For this review, use the dimensioned drawing (mm, ordinates from the lowest corner) and the shaded views. A direction names the side the tool comes from. Give positions to 0.01 mm unless a question says otherwise; leave off trailing zeros. Write each loop counter-clockwise with the first axis right and the second up, starting at its lowest first coordinate (ties: lowest second). Pieces come first, ordered by that corner, then holes. Notation, with made-up numbers: (30.25, 52) -> (49.25, 52) arc R25 ccw to (49.25, 69) -> close; hole circle Ø11 at (24, 42). An arc over 180 degrees is marked (long way). Return JSON: item names as keys, results as strings.
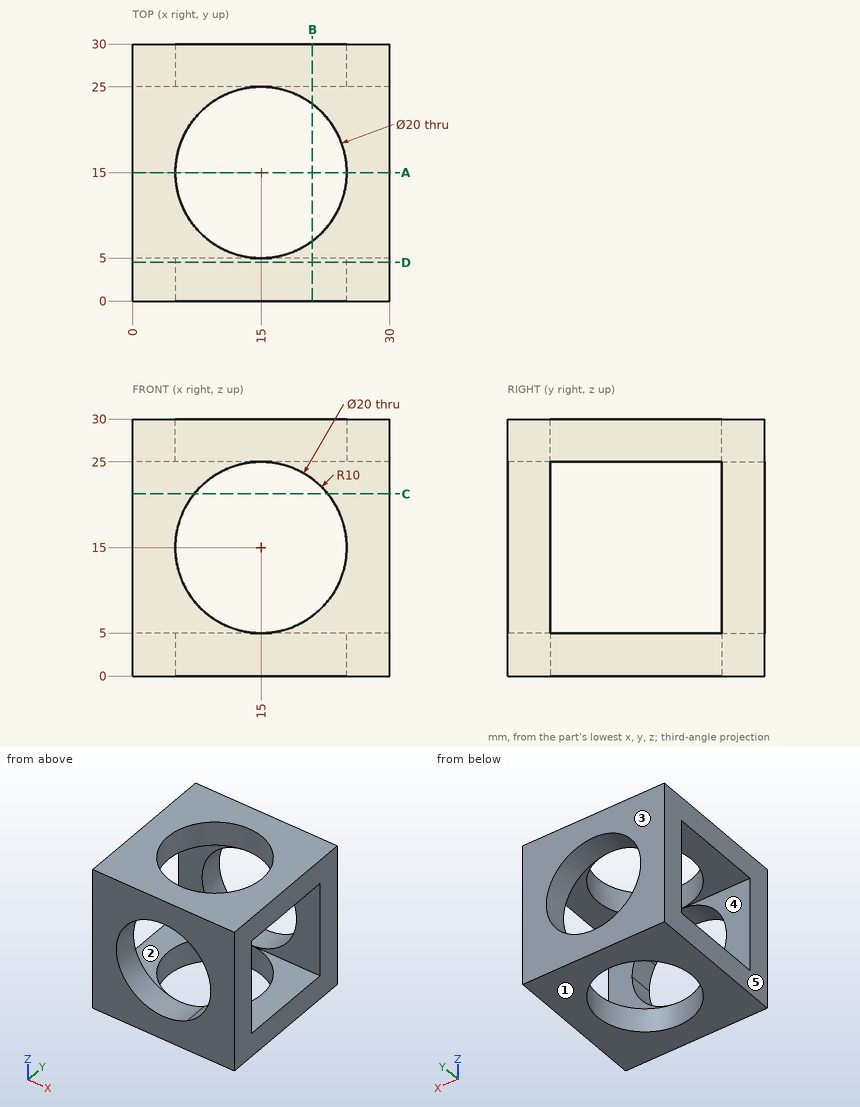
1. For pin 1 (18 mm diameter, centred on x = 15, z = 15, fed in from -Y), flat-tipped, find the tip position at first contact; note if it passes through.
Results found:
{"pin 1": "passes through"}
2. For the marked faces 4 and 5, list the 3-axis set-ups (+Z, -Z, +X, -X, +Y, -Y) from which the entire face can be reached by the end or side of a thin tool; tool diameter is ignored.
Results found:
{"face 4": "+X, -X", "face 5": "+Z, -Z, -X, +Y, -Y"}
3. The part is to be moulded in two halves that separate along Z. For the marked faces 1, 2 and 3, say which applies: +Z half, -Z half, draft (parallel to the pull), parting line (faces both ways), or undercut.
Results found:
{"face 1": "-Z half", "face 2": "undercut", "face 3": "draft"}
4. Add section A-A, the plane y = 15. State the section outline as (x, z) points, plus the area to 3 significant figures.
Results found:
{"outline": "(0, 0) -> (5, 0) -> (5, 5) -> (0, 5) -> close; (0, 25) -> (5, 25) -> (5, 30) -> (0, 30) -> close; (25, 0) -> (30, 0) -> (30, 5) -> (25, 5) -> close; (25, 25) -> (30, 25) -> (30, 30) -> (25, 30) -> close", "area": "100 mm²"}
5. To check wall thickness, follow probe 1 along Y at (x, z) = (4.25, 14.75). State the ranges of the line that lie inside material, in increasing order.
Results found:
{"probe 1": "y = 0 to 5, 25 to 30"}
6. Add section B-B, the plane x = 21. State the section outline as (y, z) points.
Results found:
{"outline": "(0, 0) -> (7, 0) -> (7, 5) -> (5, 5) -> (5, 7) -> (0, 7) -> close; (0, 23) -> (5, 23) -> (5, 25) -> (7, 25) -> (7, 30) -> (0, 30) -> close; (23, 0) -> (30, 0) -> (30, 7) -> (25, 7) -> (25, 5) -> (23, 5) -> close; (23, 25) -> (25, 25) -> (25, 23) -> (30, 23) -> (30, 30) -> (23, 30) -> close"}
7. Add section D-D, the plane y = 4.5. State the section outline as (x, z) points.
Results found:
{"outline": "(0, 0) -> (30, 0) -> (30, 30) -> (0, 30) -> close; hole circle Ø20 at (15, 15)"}
8. Add section C-C, the plane z = 21.25. State the section outline as (x, y) points.
Results found:
{"outline": "(0, 0) -> (7.19, 0) -> (7.19, 5) -> (0, 5) -> close; (0, 25) -> (7.19, 25) -> (7.19, 30) -> (0, 30) -> close; (22.81, 0) -> (30, 0) -> (30, 5) -> (22.81, 5) -> close; (22.81, 25) -> (30, 25) -> (30, 30) -> (22.81, 30) -> close"}
